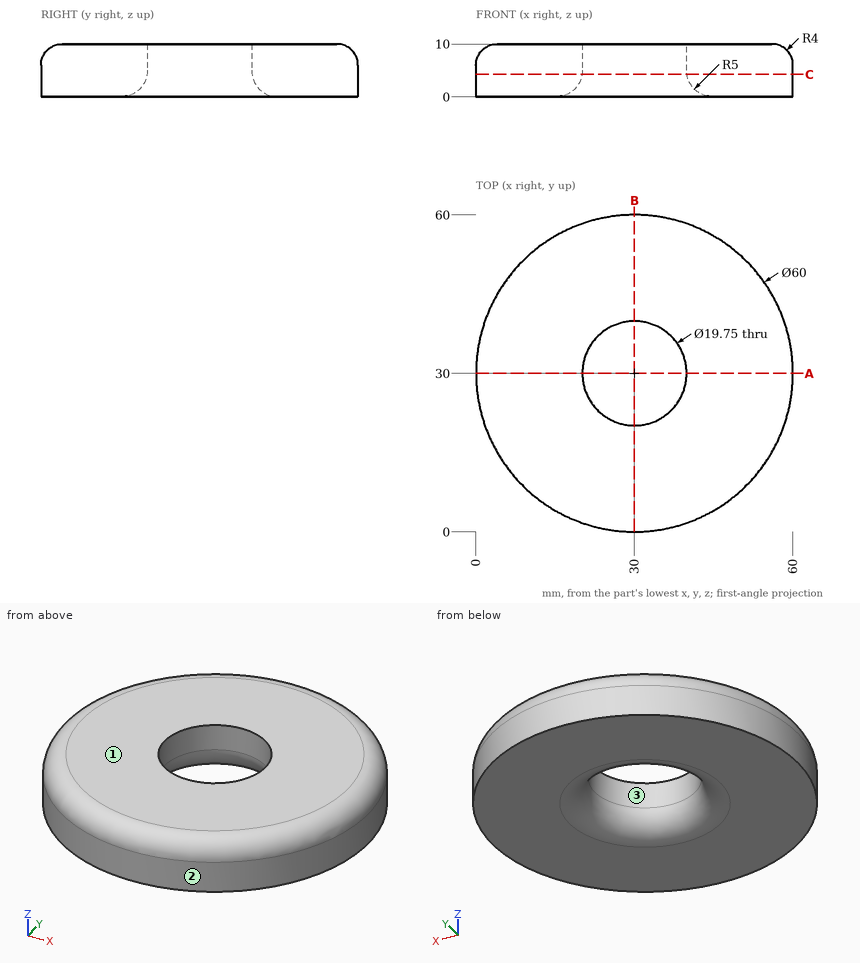
Geometry check sheet. Reference: drawing and pictorial views, mm from the part's lowest x, y, z. Give positions to 0.01 mm unless a question says otherwise; leave off trailing zeros. Loops run counter-clockwise (first coordinate to the right, second up) from the corner with the lowest first, then second, coordinate; pieces in that order, holes last. Notation, with made-up numbers: M 26.25,29.25 L 78.25,29.25 A31 ccw 78.25,53.25 Z; hole C 23,8.5 d10. An arc over 180 degrees is marked long. One line per question, with ' | ' between items.
Item 1: Draft check along X on the marked faces 1, 2 and 3. Enter one of: +X half, -X half, draft (parallel to the pull), parting line (faces both ways), or undercut.
Completed:
face 1: draft | face 2: parting line | face 3: undercut
Item 2: Section check C-C, the plane z = 4.25. Record the cut outline in (x, y).
Completed:
outline: C 30,30 d60; hole C 30,30 d19.86
Item 3: Section check A-A, the plane y = 30. Record the cut outline in (x, z) (3 decimals).
Completed:
outline: M 0,0 L 15.125,0 A5 ccw 20.125,5 L 20.125,10 L 4,10 A4 ccw 0,6 Z; M 39.875,5 A5 ccw 44.875,0 L 60,0 L 60,6 A4 ccw 56,10 L 39.875,10 Z
Item 4: Depth check by flat-ended pin: P1, Ø1.5, axis at y = 51.5, z = 7.5, coming from the +X side; P2, Ø1, axis at y = 40, z = 9, coming from the -X side; P3, Ø3, axis at y = 13.5, z = 6, coming from the -X side; P4, Ø16, axis at x = 30, y = 30, coming from the -Z side. Enter the tip coordinate at first touch or a pass-through.
Completed:
P1: stops at x = 51.35 | P2: stops at x = 2.61 | P3: stops at x = 4.02 | P4: passes through
Item 5: Thickness scan on line 1 (X direction, y = 30.5, z = 5.75); line 2 (X direction, y = 36.5, z = 6.75); line 3 (Y direction, x = 31.5, z = 2.75). Record the ranges inside material, lowest first. Write a range as [from, to].
Completed:
line 1: x = [0, 20.14], [39.86, 60] | line 2: x = [0.79, 22.57], [37.43, 59.21] | line 3: y = [0.04, 19.7], [40.3, 59.96]
